from build123d import *

# Parameters (mm, degrees)
BOSS_EXTRUDE1_DEPTH = 25.4
BOSS_EXTRUDE2_DEPTH = 3
CUT_EXTRUDE1_DEPTH  = 25.4
SKETCH3_W           = 86
SKETCH3_H           = 1.732050808
CUT_EXTRUDE2_DEPTH  = 25.4
FILLET1_SIZE        = 1.5
FILLET1_SIZE_2      = 25.4
FILLET2_R           = 6.35


# Read off the part's stored shape, not the designer's step: Cut-Extrude1
with BuildPart() as part:
    # Sketch1 → Boss-Extrude1 (new body)
    with BuildSketch(Plane(origin=(0, 0, 0), x_dir=(1, 0, 0), z_dir=(0, 1, 0))):
        Polygon((43, 24.826061575), (0, 49.65212315), (-43, 24.826061575), (-43, -24.826061575), (0, -49.65212315), (43, -24.826061575), align=None)
        Polygon((-40, -23.094010768), (0, -46.188021535), (40, -23.094010768), (40, 23.094010768), (0, 46.188021535), (-40, 23.094010768), align=None, mode=Mode.SUBTRACT)
    extrude(amount=BOSS_EXTRUDE1_DEPTH)

    # Sketch2 → Boss-Extrude2 (add)
    with BuildSketch(Plane.XZ):
        Polygon((43, 24.826061575), (0, 49.65212315), (-43, 24.826061575), (-43, -24.826061575), (0, -49.65212315), (43, -24.826061575), align=None)
    extrude(amount=BOSS_EXTRUDE2_DEPTH)

    # Cut-Extrude1 outline → Cut-Extrude1 (cut)
    with BuildSketch(Plane(origin=(0, 0, 0), x_dir=(1, 0, 0), z_dir=(0, 1, 0))):
        Polygon((40, 26.558112383), (0, 49.65212315), (-40, 26.558112383), (-40, 23.094010768), (0, 46.188021535), (40, 23.094010768), align=None)
    extrude(amount=CUT_EXTRUDE1_DEPTH, mode=Mode.SUBTRACT)

    # Sketch3 → Cut-Extrude2 (cut)
    with BuildSketch(Plane(origin=(0, 25.4, 0), x_dir=(1, 0, 0), z_dir=(0, 1, 0))):
        with Locations((0, 25.692086979)):
            Rectangle(SKETCH3_W, SKETCH3_H)
    extrude(amount=-CUT_EXTRUDE2_DEPTH, mode=Mode.SUBTRACT)

    # Fillet1
    # an asymmetric fillet: 25.4, 1.5 mm, written as the material it takes off along each edge
    with BuildSketch(Plane(origin=(40, 0, -24.826061575), x_dir=(1, 0, 0), z_dir=(0, 1, 0)), Plane(origin=(-40, 88.9, -24.826061575), x_dir=(-1, 0, 0), z_dir=(0, -1, 0))) as fillet1_piece_1:
        with BuildLine():
            Bezier((FILLET1_SIZE, 0), (0, 0), (0, -FILLET1_SIZE_2), weights=[1, 0.707106781, 1])
            Line((0, -FILLET1_SIZE_2), (0, 0))
            Line((0, 0), (FILLET1_SIZE, 0))
        make_face()
    extrude(amount=88.9, mode=Mode.SUBTRACT)

    # Fillet2
    fillet2_edges = [part.edges().sort_by_distance(p)[0] for p in [
        (-40, 12.7, 23.094010768),
        (0, 12.7, 46.188021535),
        (40, 12.7, 23.094010768),
    ]]
    fillet(fillet2_edges, radius=FILLET2_R)


solid = part.part
Input: part model. Units: mm. Frame: model coordinates. A direction names the side the tool comes from. Give positions to 0.01 mm unless a question says otherwise; leave off trailing zeros. Order: outer loops, then holes, each group sorted by start corner. A loop starts at its lowest first (then second) coordinate and runs counter-clockwise, first axis right, second up. Notation, with made-up numbers: (68.25, 49.5) -> (91.25, 49.5) arc R27 ccw to (91.25, 72.5) -> close; hole circle Ø10 at (67.25, -12). An arc over 180 degrees is marked (long way). Use one line per item in the form item = value.
1) First-contact query: pin 1 Ø10 at (x, y) = (33, 14.5) entering from +Z; pin 2 Ø2 at (x, y) = (20.5, 9.5) entering from -Z (3 decimals); pin 3 Ø5 at (x, y) = (15.5, 3.5) entering from -Z. Flat tips, straight axial feed; report the tip coordinate or a pass-through.
Response values:
pin_1 = 33.49
pin_2 = 33.775
pin_3 = 35.8
2) Section D-D, the plane x = -8.5. Return loops of the section in (y, z), and give its area (3 significant figures).
Response values:
outline = (-3, -44.74) -> (0, -44.74) -> (0, 41.28) -> (25.4, 41.28) -> (25.4, 44.74) -> (-3, 44.74) -> close
area = 356 mm^2
3) Reachability of faces 5 (the cylindrical face through (-39.172, 12.878, 22.562)), 6 (the flat face through (-21.2, 11.4, 37.41)) from +Z, -Z, +X, -X, +Y, -Y: full face, straight path, thin tool, end or side. Return the list, or none.
Response values:
face_5 = -Z, +Y
face_6 = +Z, -X, +Y, -Y
4) Section A-A, the plane z = 11. Return loops of the section in (x, y).
Response values:
outline = (-43, -3) -> (43, -3) -> (43, 25.4) -> (40, 25.4) -> (40, 0) -> (-40, 0) -> (-40, 25.4) -> (-43, 25.4) -> close
5) Section C-C, the plane z = 30. Return loops of the section in (x, y), and give its area (3 significant figures).
Response values:
outline = (-34.04, -3) -> (34.04, -3) -> (34.04, 25.4) -> (28.04, 25.4) -> (28.04, 0) -> (-28.04, 0) -> (-28.04, 25.4) -> (-34.04, 25.4) -> close
area = 509 mm^2
6) Mould query, pull axis X, two halves, no side actions, for faces 1 (the flat face through (-21.801, -1.479, -37.065)), 2 (the flat face through (21.2, -1.48, -37.41)), 3 (the flat face through (-1, -3, 1)), 4 (the flat face through (-1, 0, -3)). Classes: pulls with the +X half, pulls with the -X half, needs draft (parallel to the pull), parting line crosses it, or undercut.
Response values:
face_1 = pulls with the -X half
face_2 = pulls with the +X half
face_3 = needs draft
face_4 = undercut
7) Line query: probe 1 along X at (y, z) = (13.75, 2.5); probe 2 along Y at (x, z) = (-2, -11); probe 3 along X at (y, z) = (17, 39). Output: solid intervals per line, ascending.
Response values:
probe_1 = -43 to -40, 40 to 43
probe_2 = -3 to 0
probe_3 = -18.45 to -12.45, 12.45 to 18.45
8) Section B-B, the plane x = -20.5. Return loops of the section in (y, z), and give its area (3 significant figures).
Response values:
outline = (-3, -37.82) -> (0, -37.82) -> (0, 34.35) -> (25.4, 34.35) -> (25.4, 37.82) -> (-3, 37.82) -> close
area = 315 mm^2
